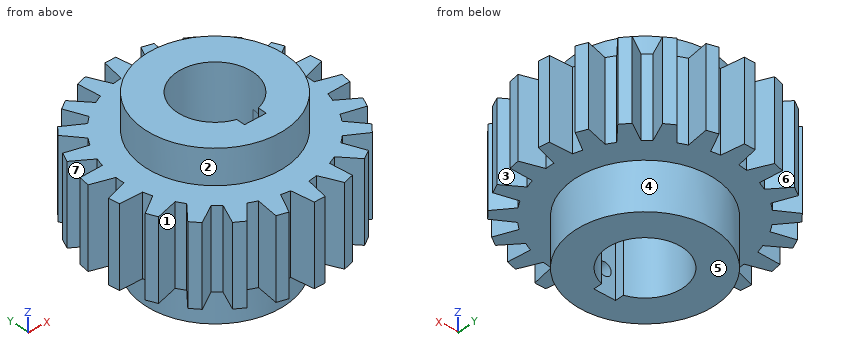
```python
from build123d import *

# Parameters (mm, degrees)
F0_R      = 43.875
F1_DEPTH  = 37
F3_DEPTH  = 37
F5_COUNT  = 22
F6_R      = 32.5
F7_DEPTH  = 22
F9_DEPTH  = 59.001
F10_R     = 3
F11_DEPTH = 33.201
F12_R     = 32.5
F13_DEPTH = 16


with BuildPart() as f1:
    # F0 (on Top) → F1 (new body)
    with BuildSketch(Plane.XY):
        Circle(F0_R)
    extrude(amount=F1_DEPTH)

    # F2 (on face) → F3 (join, through all)
    with BuildSketch(Plane.XY.offset(37)):
        with BuildLine():
            ThreePointArc((-4.2052323918, 43.6730082034), (0, 43.875), (4.2052323918, 43.6730082034))
            Line((4.2052323918, 43.6730082034), (2.5, 54))
            Line((2.5, 54), (-2.5, 54))
            Line((-2.5, 54), (-4.2052323918, 43.6730082034))
        make_face()
        with BuildLine():
            ThreePointArc((-4.2052323918, 43.6730082034), (-29.5000936762, -32.4770703435), (43.875, 0))
            ThreePointArc((43.875, 0), (32.4770703435, 29.5000936762), (4.2052323918, 43.6730082034))
            ThreePointArc((4.2052323918, 43.6730082034), (0, 43.875), (-4.2052323918, 43.6730082034))
        make_face()
    extrude(amount=-F3_DEPTH)

    # F5: F1 ×22 about axis
    f5_axis = Axis((0, 0, 35), (0, 0, 1))


with BuildPart() as f1_1:
    add(f1.part)
    for i in range(1, F5_COUNT):
        add(f1.part.rotate(f5_axis, i * 360 / F5_COUNT))

    # F6 (on face) → F7 (join)
    with BuildSketch(Plane(origin=(0, 0, 0), x_dir=(1, 0, 0), z_dir=(0, 0, -1))):
        Circle(F6_R)
    extrude(amount=F7_DEPTH)

    # F8 (on face) → F9 (cut, through all)
    with BuildSketch(Plane(origin=(0, 0, -22), x_dir=(1, 0, 0), z_dir=(0, 0, -1))):
        with BuildLine():
            Line((5, 0), (5, 16.7705098312))
            ThreePointArc((5, 16.7705098312), (0, 17.5), (-5, 16.7705098312))
            Line((-5, 16.7705098312), (-5, 0))
            Line((-5, 0), (5, 0))
        make_face()
        with BuildLine():
            ThreePointArc((-5, 16.7705098312), (0, 17.5), (5, 16.7705098312))
            Line((5, 16.7705098312), (5, 20.8))
            Line((5, 20.8), (-5, 20.8))
            Line((-5, 20.8), (-5, 16.7705098312))
        make_face()
        with BuildLine():
            ThreePointArc((-5, 16.7705098312), (-10.4582503317, -14.0312152004), (17.5, 0))
            ThreePointArc((17.5, 0), (14.0312152004, 10.4582503317), (5, 16.7705098312))
            Line((5, 16.7705098312), (5, 0))
            Line((5, 0), (-5, 0))
            Line((-5, 0), (-5, 16.7705098312))
        make_face()
    extrude(amount=-F9_DEPTH, mode=Mode.SUBTRACT)

    # F10 (on face) → F11 (cut, through all)
    with BuildSketch(Plane(origin=(0, -20.8, 0), x_dir=(-1, 0, 0), z_dir=(0, 1, 0))):
        with Locations((0, -11)):
            Circle(F10_R)
    extrude(amount=-F11_DEPTH, mode=Mode.SUBTRACT)

    # F12 (on face) → F13 (join)
    with BuildSketch(Plane.XY.offset(37)):
        Circle(F12_R)
        with BuildLine():
            ThreePointArc((-5, -16.7705098312), (0, 17.5), (5, -16.7705098312))
            Line((5, -16.7705098312), (5, -20.8))
            Line((5, -20.8), (-5, -20.8))
            Line((-5, -20.8), (-5, -16.7705098312))
        make_face(mode=Mode.SUBTRACT)
    extrude(amount=F13_DEPTH)


solid = f1_1.part
```
The model under review builds one solid part; all positions refer to its coordinate system, in mm. Face numbers are marked on the shaded views. A direction names the side the tool comes from. Round coordinates to 2 decimals unless told otherwise and drop trailing zeros. Loops run counter-clockwise (first coordinate to the right, second up) from the corner with the lowest first, then second, coordinate; pieces in that order, holes last. Notation, with made-up numbers: M -10,63.5 L 49,63.5 A19 cw 49,79.5 Z; hole C 73,-8.75 d10. An arc over 180 degrees is marked long. Answer as a JSON object with one key per item and string values.
(1) Clearance check with flat-ended pins moving along their axes: P1, Ø1.2, axis at y = -18, z = 3.5, coming from the -X side; P2, Ø1.5, axis at x = 14, z = -2, coming from the +Y side; P3, Ø5, axis at x = 0, z = -11, coming from the -Y side; P4, Ø21, axis at x = 0, y = 0, coming from the -Z side. State where each tip first meets the part, or that it passes through.
Resolved:
{"P1": "x = -47.84", "P2": "y = 29.68", "P3": "y = 17.32", "P4": "through"}
(2) To check wall thickness, follow line 1 along Y through (x, z) = (37, 26); line 2 along X through (y, z) = (-1, 25); line 3 along Y through (x, z) = (0, 29). State the ranges of each line that lie inside material, in increasing order.
Resolved:
{"line 1": "-35.92 to -26.91, -23.58 to 23.58, 26.91 to 35.92", "line 2": "-43.86 to -17.47, 17.47 to 43.86", "line 3": "-54 to -20.8, 17.5 to 54"}
(3) Draft analysis for pull direction X (two halves, no side actions). For the marked faces 5, 6 and 7, state which applies: released by +X, released by -X, zero draft, split by the parting line, or undercut.
Resolved:
{"face 5": "zero draft", "face 6": "undercut", "face 7": "released by -X"}
(4) Tool access review of the marked faces 1, 2, 3 and 4: name each direction out of +Z, -Z, +X, -X, +Y, -Y from which nothing blocks a thin tool from reaching the whole face with its end or side.
Resolved:
{"face 1": "+Z, -Z", "face 2": "+Z", "face 3": "+Z, -Z, +X", "face 4": "-Z"}
(5) Take a section at D-D on x = 24. Give the boundary of the cut face in (y, z).
Resolved:
{"outline": "M -43.36,0 L -21.91,0 L -21.91,-22 L 21.91,-22 L 21.91,0 L 43.36,0 L 43.36,37 L 21.91,37 L 21.91,53 L -21.91,53 L -21.91,37 L -43.36,37 Z"}
(6) Take a section at A-A on x = 0. Give the boundary of the cut face in (y, z), and give its area (3 significant figures).
Resolved:
{"outline": "M -54,0 L -32.5,0 L -32.5,-8 L -20.8,-8 L -20.8,53 L -32.5,53 L -32.5,37 L -54,37 Z; M -32.5,-22 L -20.8,-22 L -20.8,-14 L -32.5,-14 Z; M 17.5,-22 L 32.5,-22 L 32.5,0 L 54,0 L 54,37 L 32.5,37 L 32.5,53 L 17.5,53 Z", "area": "3,520 mm²"}
(7) Take a section at C-C on z = -11. Give the boundary of the cut face in (x, y).
Resolved:
{"outline": "M -5,-20.8 L -5,-16.77 A17.5 cw long 5,-16.77 L 5,-20.8 L 3,-20.8 L 3,-32.36 A32.5 ccw long -3,-32.36 L -3,-20.8 Z"}
(8) Take a section at B-B on y = 3.5. Give the boundary of the cut face in (x, z), and give its area (3 significant figures).
Resolved:
{"outline": "M -48.4,0 L -32.31,0 L -32.31,-22 L -17.15,-22 L -17.15,53 L -32.31,53 L -32.31,37 L -48.4,37 Z; M 17.15,-22 L 32.31,-22 L 32.31,0 L 48.4,0 L 48.4,37 L 32.31,37 L 32.31,53 L 17.15,53 Z", "area": "3,470 mm²"}
